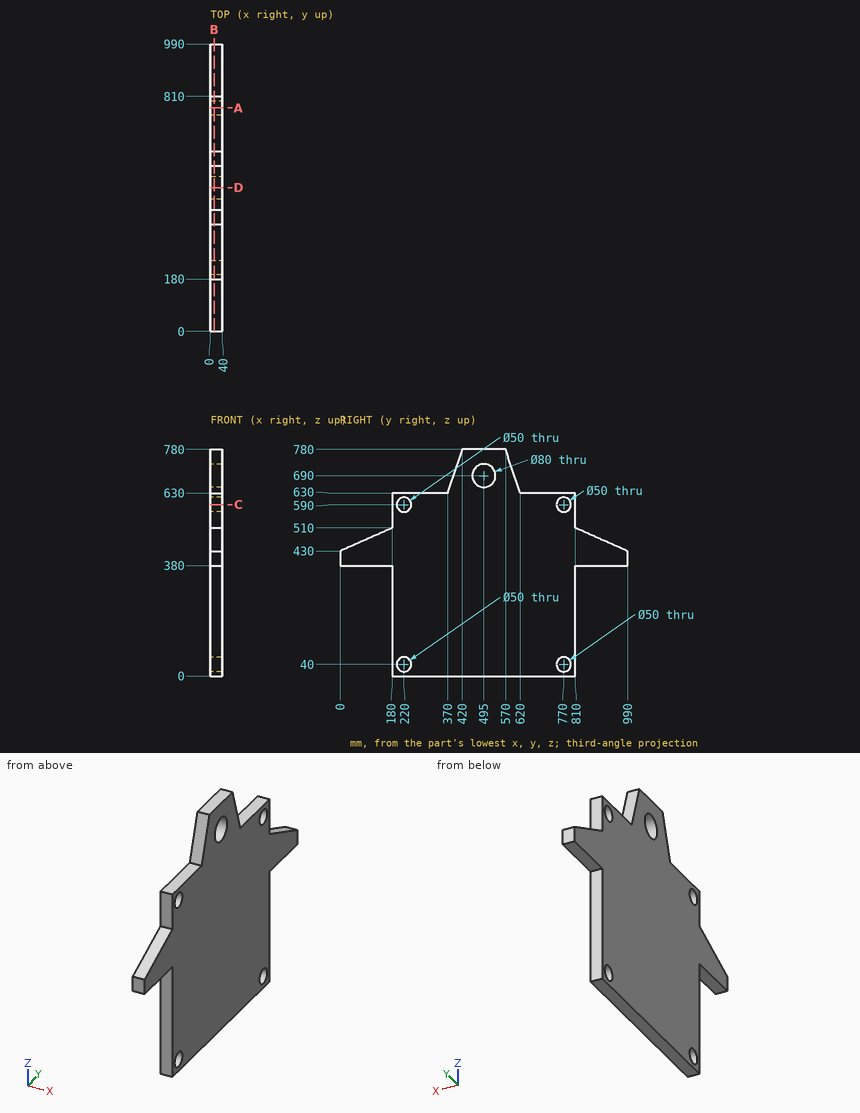
Can you work these out from the drawing? Everything is in mm from the part's minimum corner. Round coordinates to 2 decimals unless told otherwise and drop trailing zeros. Order: outer loops, then holes, each group sorted by start corner. A loop starts at its lowest first (then second) coordinate and runs counter-clockwise, first axis right, second up. Notation, with made-up numbers: (0, 39) -> (44, 39) arc R6 cw to (44, 46) -> close; hole circle Ø5 at (76.5, 58.5). An arc over 180 degrees is marked (long way). Use CSV: the item, a comma, the result in double quotes.
1. I want a section at A-A on y = 770. List the corners of the cut face in (x, z) for me, and give its area (3 significant figures).
Recorded:
outline,"(0, 0) -> (40, 0) -> (40, 15) -> (0, 15) -> close; (0, 65) -> (40, 65) -> (40, 565) -> (0, 565) -> close; (0, 615) -> (40, 615) -> (40, 630) -> (0, 630) -> close"
area,"21,200 mm2"
2. I want a section at D-D on y = 495. List the corners of the cut face in (x, z) for me, and give its area (3 significant figures).
Recorded:
outline,"(0, 0) -> (40, 0) -> (40, 650) -> (0, 650) -> close; (0, 730) -> (40, 730) -> (40, 780) -> (0, 780) -> close"
area,"28,000 mm2"
3. I want a section at C-C on z = 590. List the corners of the cut face in (x, y) for me, and give its area (3 significant figures).
Recorded:
outline,"(0, 180) -> (40, 180) -> (40, 195) -> (0, 195) -> close; (0, 245) -> (40, 245) -> (40, 745) -> (0, 745) -> close; (0, 795) -> (40, 795) -> (40, 810) -> (0, 810) -> close"
area,"21,200 mm2"
4. I'm going to push flat-ended pins straight in: P1, Ø12, axis at x = 10.5, z = 241.5, coming from the +Y side; P2, Ø2, axis at x = 10.5, z = 394, coming from the -Y side; P3, Ø20, axis at x = 12.5, z = 594, coming from the -Y side; P4, Ø20, axis at x = 16, y = 112, coming from the -Z side. Where does each tip first touch, or does it pass through?
Recorded:
P1,"stops at y = 810"
P2,"stops at y = 0"
P3,"stops at y = 180"
P4,"stops at z = 380"
5. I need wall thicknesses on line 1 along Z through (x, y) = (23, 220); line 2 along Y through (x, z) = (25, 123); line 3 along Y through (x, z) = (14.5, 688.5). Which ranges of each line are inside material? Lowest first, please.
Recorded:
line 1,"z = 0 to 15, 65 to 565, 615 to 630"
line 2,"y = 180 to 810"
line 3,"y = 389.5 to 455.03, 534.97 to 600.5"
6. I want a section at B-B on x = 12.5. List the corners of the cut face in (y, z) for me, and give its area (3 significant figures).
Recorded:
outline,"(0, 380) -> (180, 380) -> (180, 0) -> (810, 0) -> (810, 380) -> (990, 380) -> (990, 430) -> (810, 510) -> (810, 630) -> (620, 630) -> (570, 780) -> (420, 780) -> (370, 630) -> (180, 630) -> (180, 510) -> (0, 430) -> close; hole circle Ø50 at (220, 40); hole circle Ø50 at (220, 590); hole circle Ø80 at (495, 690); hole circle Ø50 at (770, 40); hole circle Ø50 at (770, 590)"
area,"446,000 mm2"
